```python
from build123d import *

# Parameters (mm, degrees)
SKETCH1_R               = 2.25
BOSS_EXTRUDE1_DEPTH     = 19.05
SKETCH2_W               = 16.825
SKETCH2_H               = 3.275
CUT_EXTRUDE1_DEPTH      = 20.725
CUT_EXTRUDE1_DEPTH_BACK = 20.725
SKETCH4_R               = 2.25
CUT_EXTRUDE2_DEPTH      = 30.725
CUT_EXTRUDE2_DEPTH_BACK = 20.725


with BuildPart() as part:
    # Sketch1 → Boss-Extrude1 (new body, symmetric)
    with BuildSketch(Plane.XY):
        with BuildLine():
            Line((-9.725, 9.725), (-14.725, 9.725))
            ThreePointArc((-14.725, 9.725), (-18.260533906, 8.260533906), (-19.725, 4.725))
            Line((-19.725, 4.725), (-19.725, -14.725))
            ThreePointArc((-19.725, -14.725), (-18.260533906, -18.260533906), (-14.725, -19.725))
            Line((-14.725, -19.725), (24.725, -19.725))
            ThreePointArc((24.725, -19.725), (28.260533906, -18.260533906), (29.725, -14.725))
            Line((29.725, -14.725), (29.725, 14.725))
            ThreePointArc((29.725, 14.725), (28.260533906, 18.260533906), (24.725, 19.725))
            Line((24.725, 19.725), (9.725, 19.725))
            Line((9.725, 19.725), (9.725, 9.725))
            Line((9.725, 9.725), (9.725, -9.725))
            Line((9.725, -9.725), (-9.725, -9.725))
            Line((-9.725, -9.725), (-9.725, 9.725))
        make_face()
        with Locations((19.725, 12.5)):
            Circle(SKETCH1_R, mode=Mode.SUBTRACT)
        with Locations((19.725, -12.5)):
            Circle(SKETCH1_R, mode=Mode.SUBTRACT)
    extrude(amount=BOSS_EXTRUDE1_DEPTH, both=True)

    # Sketch2 → Cut-Extrude1 (cut, two sides)
    with BuildSketch(Plane(origin=(0, 0, 0), x_dir=(1, 0, 0), z_dir=(0, 1, 0))) as cut_extrude1_sk:
        with Locations((21.3125, 14.3375)):
            Rectangle(SKETCH2_W, SKETCH2_H)
        with Locations((21.3125, -14.3375)):
            Rectangle(SKETCH2_W, SKETCH2_H)
    extrude(amount=CUT_EXTRUDE1_DEPTH, mode=Mode.SUBTRACT)
    extrude(cut_extrude1_sk.sketch, amount=-CUT_EXTRUDE1_DEPTH_BACK, mode=Mode.SUBTRACT)

    # Sketch4 → Cut-Extrude2 (cut, two sides)
    with BuildSketch(Plane(origin=(0, 0, 0), x_dir=(0, 0, -1), z_dir=(1, 0, 0))) as cut_extrude2_sk:
        with Locations((-6.35, 0)):
            Circle(SKETCH4_R)
        with Locations((6.35, 0)):
            Circle(SKETCH4_R)
    extrude(amount=CUT_EXTRUDE2_DEPTH, mode=Mode.SUBTRACT)
    extrude(cut_extrude2_sk.sketch, amount=-CUT_EXTRUDE2_DEPTH_BACK, mode=Mode.SUBTRACT)


solid = part.part
```
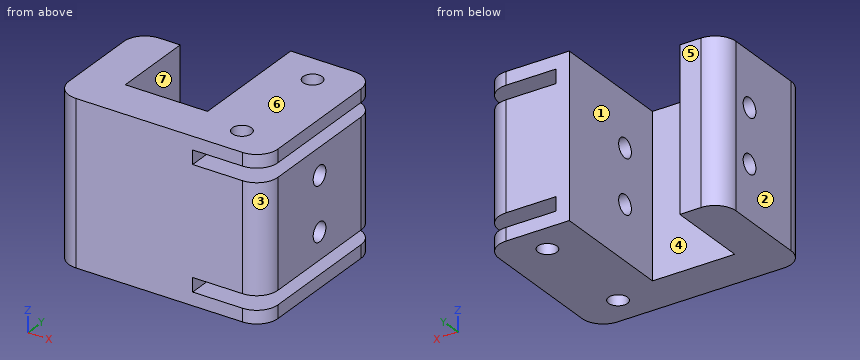
Geometry: final body of the model. Coordinates: model frame, mm. Face numbers are marked on the shaded views. A direction names the side the tool comes from. Coordinates: 2 decimals unless noted, no trailing zeros. Order: outer loops, then holes, each group sorted by start corner. A loop starts at its lowest first (then second) coordinate and runs counter-clockwise, first axis right, second up. Notation, with made-up numbers: M -17.75,4.5 L -12.75,4.5 A13 cw -12.75,25.5 Z; hole C -15,-12.75 d2. An arc over 180 degrees is marked long. Answer in a Markdown table with one row per item. Add a question column.
Q1. Mould query, pull axis X, two halves, no side actions, for the marked faces 1, 2, 3 and 4. Classes: released by +X, released by -X, zero draft, split by the parting line, or undercut.
Q2. Section query C-C on y = -12.5. Return the cut outline in (x, z) (3 decimals).
Q3. Section query B-B on z = -5.5. Return the cut outline in (x, y) (3 decimals).
Q4. Section query D-D on y = 0. Count the separate pieces of the cut face and the enclosed holes in it, and give its area (3 significant figures).
Q5. Line query: L1, parallel to Z at x = 18, y = 9 (3 decimals); L2, parallel to Z at x = 18.5, y = 0 (3 decimals); L3, parallel to Z at x = -12, y = -2. Output: solid intervals per line, ascending.
Q6. Section query A-A on x = 24. Return the cut outline in (y, z) (3 decimals).
Q7. Contact query for flat-ended pins moving along their axis: P1, Ø12, axis at x = 2, z = 5, coming from the +Y side (3 decimals); P2, Ø1.5, axis at x = -13, z = -2.5, coming from the +Y side (3 decimals); P3, Ø1.6, axis at y = -9, z = -15, coming from the +X side. Output: stop coordinate, or through.
Q8. Reachability of the marked faces 5, 6 and 7 from +Z, -Z, +X, -X, +Y, -Y: full face, straight path, thin tool, end or side. Return the list, or none.
Completed:
| question | item | result |
|---|---|---|
| 1 | face 1 | undercut |
| 1 | face 2 | released by -X |
| 1 | face 3 | released by +X |
| 1 | face 4 | undercut |
| 2 | outline | M -19.725,-19.05 L 17.475,-19.05 L 17.475,-15.975 L 12.9,-15.975 L 12.9,-12.7 L 17.475,-12.7 L 17.475,12.7 L 12.9,12.7 L 12.9,15.975 L 17.475,15.975 L 17.475,19.05 L -19.725,19.05 Z; M 21.975,-19.05 L 29.725,-19.05 L 29.725,-15.975 L 21.975,-15.975 Z; M 21.975,-12.7 L 29.725,-12.7 L 29.725,12.7 L 21.975,12.7 Z; M 21.975,15.975 L 29.725,15.975 L 29.725,19.05 L 21.975,19.05 Z |
| 3 | outline | M -19.725,-14.725 A5 ccw -14.725,-19.725 L 24.725,-19.725 A5 ccw 29.725,-14.725 L 29.725,-2.083 L 9.725,-2.083 L 9.725,-9.725 L -9.725,-9.725 L -9.725,-2.083 L -19.725,-2.083 Z; M -19.725,2.083 L -9.725,2.083 L -9.725,9.725 L -14.725,9.725 A5 ccw -19.725,4.725 Z; M 9.725,2.083 L 29.725,2.083 L 29.725,14.725 A5 ccw 24.725,19.725 L 9.725,19.725 Z; hole C 19.725,-12.5 d4.5; hole C 19.725,12.5 d4.5 |
| 4 | separate pieces | 6 |
| 4 | enclosed holes | 0 |
| 4 | area | 763 mm2 |
| 5 | L1 | z = -19.05 to -15.975, -12.7 to 12.7, 15.975 to 19.05 |
| 5 | L2 | z = -19.05 to -15.975, -12.7 to -8.6, -4.1 to 4.1, 8.6 to 12.7, 15.975 to 19.05 |
| 5 | L3 | z = -19.05 to -7.38, -5.32 to 5.32, 7.38 to 19.05 |
| 6 | outline | M -19.725,-19.05 L 19.725,-19.05 L 19.725,-15.975 L -19.725,-15.975 Z; M -19.725,-12.7 L 19.725,-12.7 L 19.725,12.7 L -19.725,12.7 Z; M -19.725,15.975 L 19.725,15.975 L 19.725,19.05 L -19.725,19.05 Z; hole C 0,-6.35 d4.5; hole C 0,6.35 d4.5 |
| 7 | P1 | stops at y = -9.725 |
| 7 | P2 | stops at y = 9.725 |
| 7 | P3 | stops at x = 12.9 |
| 8 | face 5 | +Z, -Z, -X, +Y |
| 8 | face 6 | +Z, +X, -X, +Y, -Y |
| 8 | face 7 | +Z, -Z, +Y |
